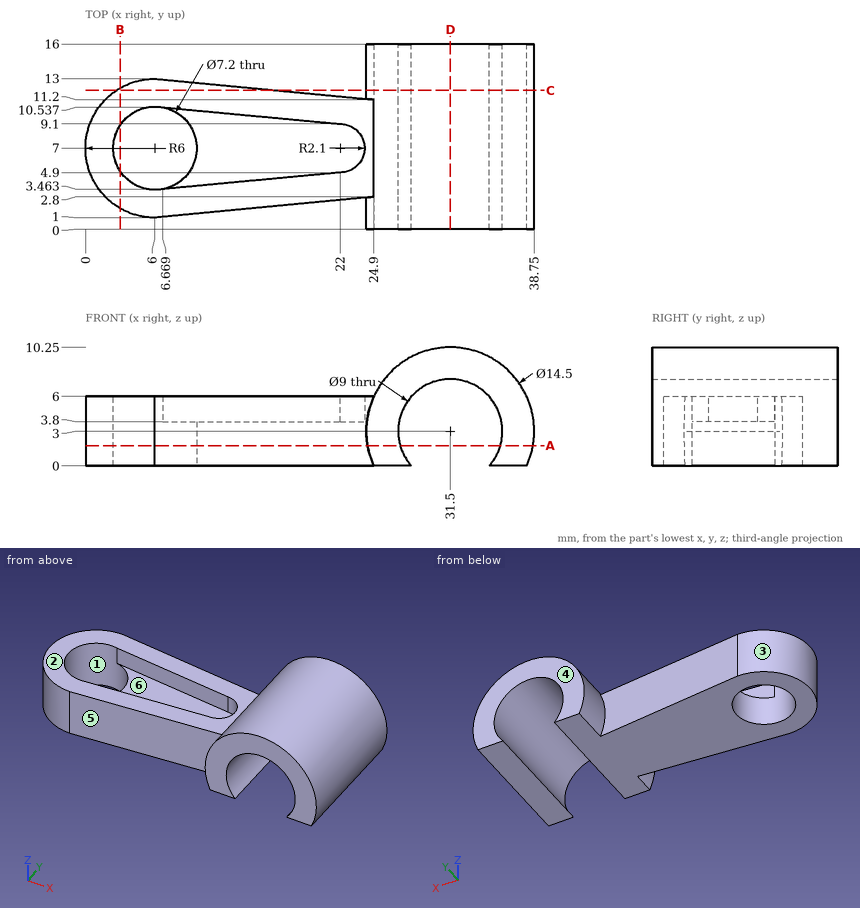
Geometry check sheet. Reference: drawing and pictorial views, mm from the part's lowest x, y, z. A direction names the side the tool comes from. Round coordinates to 2 decimals unless told otherwise and drop trailing zeros. Order: outer loops, then holes, each group sorted by start corner. A loop starts at its lowest first (then second) coordinate and runs counter-clockwise, first axis right, second up.
Q1. Set-up check for the marked faces 1 and 2: record each of +Z, -Z, +X, -X, +Y, -Y from which the full face is reachable in a straight line by a thin tool's end or side.
Filled sheet:
face 1: +Z, -Z
face 2: +Z, -X, +Y, -Y
Q2. Cross-section at C-C, the plane y = 12. Enter the section's corners in (x, z), plus the area to 3 significant figures.
Filled sheet:
outline: (2.68, 0) - (16.5, 0) - (16.5, 6) - (2.68, 6) - close; (24.9, 0) - (28.15, 0) arc R4.5 cw (long way) to (34.85, 0) - (38.1, 0) arc R7.25 ccw (long way) to start
area: 151 mm2
Q3. Cross-section at B-B, the plane x = 3. Enter the section's corners in (y, z).
Filled sheet:
outline: (1.8, 0) - (5.01, 0) - (5.01, 6) - (1.8, 6) - close; (8.99, 0) - (12.2, 0) - (12.2, 6) - (8.99, 6) - close
Q4. Scan lines: L1, parallel to X at y = 7, z = 3.1; L2, parallel to Y at x = 6, z = 1.35; L3, parallel to X at y = 5.5, z = 3.5. Record each from-to range of solid material in increasing order.
Filled sheet:
L1: x = 0 to 2.4, 9.6 to 27, 36 to 38.75
L2: y = 1 to 3.4, 10.6 to 13
L3: x = 0.19 to 2.73, 9.27 to 27.03, 35.97 to 38.73
Q5. Draft check along X on the marked faces 3, 4, 5 and 6. Enter one of: pulls with the +X half, pulls with the -X half, needs draft (parallel to the pull), parting line crosses it, or undercut.
Filled sheet:
face 3: pulls with the -X half
face 4: needs draft
face 5: undercut
face 6: undercut
Q6. Depth check by flat-ended pin: P1, Ø1, axis at y = 4.5, z = 1, coming from the +X side; P2, Ø4, axis at x = 32.5, y = 9.5, coming from the -Z side (1 decimal); P3, Ø3.5, axis at x = 10, y = 5, coming from the +Z side. Enter the tip coordinate at first touch or a pass-through.
Filled sheet:
P1: stops at x = 38.59
P2: stops at z = 6.4
P3: stops at z = 6
Q7. Cross-section at D-D, the plane x = 31.5. Enter the section's corners in (y, z), plus the area to 3 significant figures.
Filled sheet:
outline: (0, 7.5) - (16, 7.5) - (16, 10.25) - (0, 10.25) - close
area: 44.0 mm2
Q8. Cross-section at A-A, the plane z = 1.75. Enter the section's corners in (x, y).
Filled sheet:
outline: (6, 1) - (24.36, 2.75) - (24.36, 0) - (27.18, 0) - (27.18, 16) - (24.36, 16) - (24.36, 11.25) - (6, 13) arc R6 ccw to start; (35.82, 0) - (38.64, 0) - (38.64, 16) - (35.82, 16) - close; hole circle Ø7.2 at (6, 7)
